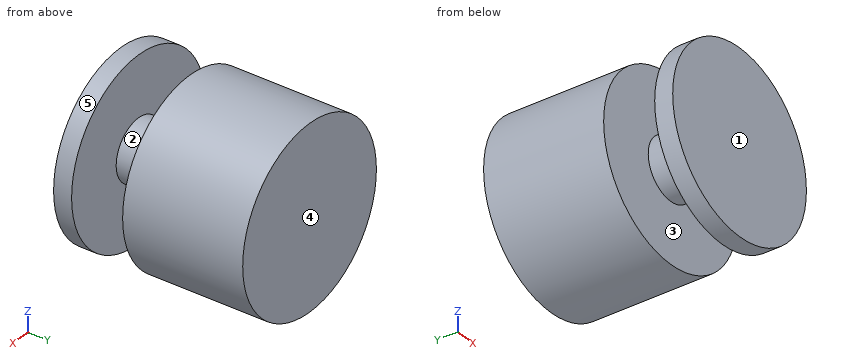
Autodesk Inventor part; units mm, degrees
ref_plane "YZ Plane" through (0, 0, 0) normal (1, 0, 0) x (0, 1, 0)
ref_plane "XZ Plane" through (0, 0, 0) normal (0, 1, 0) x (-1, 0, 0)
ref_plane "XY Plane" through (0, 0, 0) normal (0, 0, 1) x (1, 0, 0)
sketch "Sketch1" plane through (0, 0, 0) normal (1, 0, 0) x (0, 1, 0)
  line L0 (-12.7, 6.35) -> (12.7, 6.35)
  line L1 (12.7, 6.35) -> (12.7, -6.35)
  line L2 (12.7, -6.35) -> (-12.7, -6.35)
  line L3 (-12.7, -6.35) -> (-12.7, 6.35)
  line L4 (-12.7, 6.35) -> (12.7, -6.35) construction
  line L5 (12.7, 6.35) -> (-12.7, -6.35) construction
  line L6 (-14.605, 19.05) -> (-10.795, 19.05)
  line L7 (-10.795, 19.05) -> (-10.795, -19.05)
  line L8 (-10.795, -19.05) -> (-14.605, -19.05)
  line L9 (-14.605, -19.05) -> (-14.605, 19.05)
  line L10 (-14.605, 19.05) -> (-10.795, -19.05) construction
  line L11 (-10.795, 19.05) -> (-14.605, -19.05) construction
  line L12 (0, 19.05) -> (25.4, 19.05)
  line L13 (25.4, 19.05) -> (25.4, -19.05)
  line L14 (25.4, -19.05) -> (0, -19.05)
  line L15 (0, -19.05) -> (0, 19.05)
  line L16 (0, 19.05) -> (25.4, -19.05) construction
  line L17 (25.4, 19.05) -> (0, -19.05) construction
  line L18 (-14.605, 0) -> (25.4, 0)
  point P0 (0, 0)
  point P1 (-12.7, 0)
  point P2 (12.7, 0)
  point P3 (-10.795, -6.35)
  point P4 (0, -6.35)
  dimension "d0" = 25.4
  dimension "d1" = 38.1
  dimension "d2" = 3.81
  dimension "d3" = 38.1
  dimension "d5" = 25.4
  dimension "d6" = 12.7
revolve "Revolution1" add sketch "Sketch1" angle 360 about axis through (0, -14.605, 0) along (0, 1, 0) contours L18 L7 L2 L3 | L3 L2 L7 L8 L9 L18 | L18 L15 L2 L7 | L18 L1 L2 L15 | L18 L13 L14 L15 L2 L1
sketch "Sketch2" plane through (0, 25.4, 0) normal (0, 1, 0) x (1, 0, 0)
  point P0 (0, 0)
properties part number "pallet"
Check sheet for the modelled part. Datum: model origin and axes. Units: mm. Face numbers are marked on the shaded views. A direction names the side the tool comes from. Round coordinates to 2 decimals unless told otherwise and drop trailing zeros. Write each loop counter-clockwise with the first axis right and the second up, starting at its lowest first coordinate (ties: lowest second). Pieces come first, ordered by that corner, then holes. Notation, with made-up numbers: (33.25, 73.5) -> (41.25, 73.5) arc R31 ccw to (41.25, 107.5) -> close; hole circle Ø8 at (42, 65.5). An arc over 180 degrees is marked (long way). Put each result on its own line as item: value.
(1) Sectioned sample at C-C (x = 7.5). Enter the section's corners in (y, z) (1 decimal), plus the area to 3 significant figures.
Values found:
outline: (-14.6, -17.5) -> (-10.8, -17.5) -> (-10.8, 17.5) -> (-14.6, 17.5) -> close; (0, -17.5) -> (25.4, -17.5) -> (25.4, 17.5) -> (0, 17.5) -> close
area: 1,020 mm^2
(2) Sectioned sample at B-B (z = 0). Enter the section's corners in (x, y) (3 decimals), plus the area to 3 significant figures.
Values found:
outline: (-19.05, -14.605) -> (19.05, -14.605) -> (19.05, -10.795) -> (6.35, -10.795) -> (6.35, 0) -> (19.05, 0) -> (19.05, 25.4) -> (-19.05, 25.4) -> (-19.05, 0) -> (-6.35, 0) -> (-6.35, -10.795) -> (-19.05, -10.795) -> close
area: 1,250 mm^2
(3) Sectioned sample at D-D (y = 1.5). Enter the section's corners in (x, z), plus the area to 3 significant figures.
Values found:
outline: circle Ø38.1 at (0, 0)
area: 1,140 mm^2
(4) Material ranges on line 1 (Y direction, x = 6, z = 12) (3 decimals); line 2 (X direction, y = 20, z = 13); line 3 (X direction, y = 13.5, z = -2), recorded low to high.
Values found:
line 1: y = -14.605 to -10.795, 0 to 25.4
line 2: x = -13.92 to 13.92
line 3: x = -18.94 to 18.94
(5) Sectioned sample at A-A (x = 0). Enter the section's corners in (y, z) (3 decimals), plus the area to 3 significant figures.
Values found:
outline: (-14.605, -19.05) -> (-10.795, -19.05) -> (-10.795, -6.35) -> (0, -6.35) -> (0, -19.05) -> (25.4, -19.05) -> (25.4, 19.05) -> (0, 19.05) -> (0, 6.35) -> (-10.795, 6.35) -> (-10.795, 19.05) -> (-14.605, 19.05) -> close
area: 1,250 mm^2
(6) Mould release check, pull along Y, two halves, no side actions. Record for the marked faces 3, 4 and 5: released by +Y, released by -Y, zero draft, split by the parting line, or undercut.
Values found:
face 3: undercut
face 4: released by +Y
face 5: zero draft
(7) Tool access check on the marked faces 1 and 2. Record the directions out of +Z, -Z, +X, -X, +Y, -Y that give a thin tool (end or side, any length) a straight path to the whole face; none if there is none.
Values found:
face 1: +Z, -Z, +X, -X, -Y
face 2: none
(8) Go/stop test with flat-tipped pins: pin 1 Ø5 at (y, z) = (10, -2.5) entering from -X; pin 2 Ø2 at (x, y) = (8.5, 10) entering from -Z; pin 3 Ø5 at (x, y) = (14, 10.5) entering from +Z. Record where each tip stops, or that it passes through.
Values found:
pin 1: stops at x = -19.05
pin 2: stops at z = -17.51
pin 3: stops at z = 15.19
